```python
from build123d import *

# Parameters (mm, degrees)
F0_R          = 12.7
F1_DEPTH      = 609.6
F1_DEPTH_BACK = 609.6
F3_R          = 12.7
F8_R          = 12.7


# Not quite as in the source:
# - a pattern or mirror of a feature is missing from the dataset's text; its kind, count and spacing are read off the source's solid


with BuildPart() as f1:
    # F0 (on Front) → F1 (new body, two sides)
    with BuildSketch(Plane.XZ) as f1_sk:
        Circle(F0_R)
    extrude(amount=F1_DEPTH)
    extrude(f1_sk.sketch, amount=-F1_DEPTH_BACK)

    # F5: sweep along a path in F4
    with BuildLine(Plane.YZ) as f5_path:
        ThreePointArc((609.6, 0), (627.5605122421, 7.4394877579), (635, 25.4))
        Line((635, 25.4), (635, 38.1))
    # F3 (on offset) → F5 (sweep)
    with BuildSketch(Plane.XY.offset(38.1)):
        with Locations((0, 635)):
            Circle(F3_R)
    f5 = sweep(path=f5_path.line)

    # F5_copies: F5 across plane
    add(f5.mirror(Plane(origin=(0, 0, 0), x_dir=(0, 0, -1), z_dir=(0, -1, 0))))

    # F8 (on offset) → F9 (join, up to the next surface of F1)
    with BuildSketch(Plane.XY.offset(38.1)):
        with Locations((0, 304.8)):
            Circle(F8_R)
        with Locations((0, -304.8)):
            Circle(F8_R)
        Circle(F8_R)
    extrude(until=Until.NEXT, dir=(0, 0, -1))


solid = f1.part
```
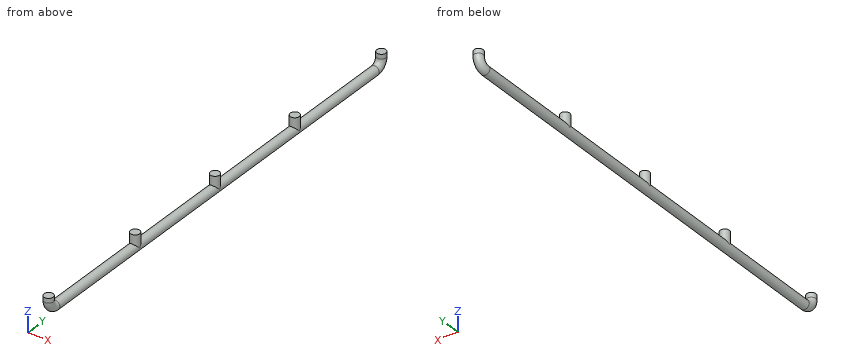
Check sheet for the modelled part. Datum: model origin and axes. Units: mm. Give positions to 0.01 mm unless a question says otherwise; leave off trailing zeros. Write each loop counter-clockwise with the first axis right and the second up, starting at its lowest first coordinate (ties: lowest second). Pieces come first, ordered by that corner, then holes. Notation, with made-up numbers: (76.25, 22) -> (117.25, 22) arc R36 ccw to (117.25, 60) -> close; hole circle Ø7 at (1.25, 60.25). An arc over 180 degrees is marked (long way). Use CSV: the item, a comma, the result in double quotes. Start each with the question number.
Q1. Depth check by flat-ended pin: P1, Ø12, axis at y = -351.5, z = 11, coming from the +X side; P2, Ø4, axis at x = -2, z = 6, coming from the +Y side; P3, Ø4, axis at x = -7, z = 21, coming from the +Y side. Enter the tip coordinate at first touch or a pass-through.
Q2. Cross-section at B-B on y = -379. Enter the section's corners in (x, z).
Q3. Cross-section at A-A on x = 0. Enter the section's corners in (y, z), and give its area (3 significant figures).
Q4. Cross-section at C-C on y = 304.8. Enter the section's corners in (x, z).
Q5. Scan lines: line 1 along Y through (x, z) = (-0.25, 30); line 2 along Y through (x, z) = (1.5, 34); line 3 along Z through (x, y) = (-1.75, -226). Record each from-to range of solid material in increasing order.
Working result:
1,P1,"stops at x = 11.67"
1,P2,"stops at y = 643.36"
1,P3,"stops at y = 646.44"
2,outline,"circle Ø25.4 at (0, 0)"
3,outline,"(-647.7, 25.4) arc R38.1 ccw to (-609.6, -12.7) -> (609.6, -12.7) arc R38.1 ccw to (647.7, 25.4) -> (647.7, 38.1) -> (622.3, 38.1) -> (622.3, 25.4) arc R12.7 cw to (609.6, 12.7) -> (317.5, 12.7) -> (317.5, 38.1) -> (292.1, 38.1) -> (292.1, 12.7) -> (12.7, 12.7) -> (12.7, 38.1) -> (-12.7, 38.1) -> (-12.7, 12.7) -> (-292.1, 12.7) -> (-292.1, 38.1) -> (-317.5, 38.1) -> (-317.5, 12.7) -> (-609.6, 12.7) arc R12.7 cw to (-622.3, 25.4) -> (-622.3, 38.1) -> (-647.7, 38.1) -> close"
3,area,"35,600 mm^2"
4,outline,"(-12.7, 0) arc R12.7 ccw to (12.7, 0) -> (12.7, 38.1) -> (-12.7, 38.1) -> close"
5,line 1,"y = -647.7 to -622.3, -317.5 to -292.1, -12.7 to 12.7, 292.1 to 317.5, 622.3 to 647.7"
5,line 2,"y = -647.61 to -622.39, -317.41 to -292.19, -12.61 to 12.61, 292.19 to 317.41, 622.39 to 647.61"
5,line 3,"z = -12.58 to 12.58"
